CAD build for the part. Positions are in the model's coordinates, mm. A direction names the side the tool comes from. Coordinates: 2 decimals unless noted, no trailing zeros. Order: outer loops, then holes, each group sorted by start corner. A loop starts at its lowest first (then second) coordinate and runs counter-clockwise, first axis right, second up. Notation, with made-up numbers: (45, 83) - (93, 83) arc R15 cw to (93, 108) - close; hole circle Ø6 at (-1, 29). An arc over 180 degrees is marked (long way). Return JSON: item names as keys, results as strings.
from build123d import *

# Parameters (mm, degrees)
SKETCH1_R           = 5.55625
BOSS_EXTRUDE1_DEPTH = 12.7
BOSS_EXTRUDE2_DEPTH = 11.938


with BuildPart() as part:
    # Sketch1 → Boss-Extrude1 (new body)
    with BuildSketch(Plane(origin=(0, 0, 0), x_dir=(1, 0, 0), z_dir=(0, 1, 0))):
        Circle(SKETCH1_R)
    extrude(amount=BOSS_EXTRUDE1_DEPTH)

    # Sketch3 → Boss-Extrude2 (add)
    with BuildSketch(Plane(origin=(0, 12.7, 0), x_dir=(1, 0, 0), z_dir=(0, 1, 0))):
        Polygon((-10.287, 1.232393343), (-10.287, -1.232393343), (-6.210783894, -8.292606741), (-4.076216154, -9.525), (4.076216154, -9.525), (6.210783894, -8.292606741), (10.287, -1.232393343), (10.287, 1.232393343), (6.210783894, 8.292606741), (4.076216154, 9.525), (-4.076216154, 9.525), (-6.210783894, 8.292606741), align=None)
    extrude(amount=BOSS_EXTRUDE2_DEPTH)


solid = part.part
Item 1: Which spindle directions (+Z, -Z, +X, -X, +Y, -Y) get a long thin tool onto all of the face, cutting with end or side? Do faces 1 (the flat face through (-5, 12.7, -4)), 2 (the flat face through (0, 0, 0)). Say none if no direction does.
Findings below:
{"face 1": "-Y", "face 2": "+Z, -Z, +X, -X, -Y"}
Item 2: Band-saw the part on C-C, the plane x = 0. List the corners of the cut face in (y, z) (3 decimals).
Findings below:
{"outline": "(0, -5.556) - (12.7, -5.556) - (12.7, -9.525) - (24.638, -9.525) - (24.638, 9.525) - (12.7, 9.525) - (12.7, 5.556) - (0, 5.556) - close"}
Item 3: Band-saw the part on B-B, the plane y = 21.75. List the corners of the cut face in (x, z) (3 decimals).
Findings below:
{"outline": "(-10.287, -1.232) - (-6.211, -8.293) - (-4.076, -9.525) - (4.076, -9.525) - (6.211, -8.293) - (10.287, -1.232) - (10.287, 1.232) - (6.211, 8.293) - (4.076, 9.525) - (-4.076, 9.525) - (-6.211, 8.293) - (-10.287, 1.232) - close"}
Item 4: Band-saw the part on D-D, the plane y = 10.5. List the corners of the cut face in (x, z), then the cut area to 3 significant figures.
Findings below:
{"outline": "circle Ø11.11 at (0, 0)", "area": "97.0 mm²"}
Item 5: Drop flat-ended pins along their axis: P1, Ø6, axis at y = 12, z = -7.5, coming from the -X side; P2, Ø2, axis at x = -4, y = 3.5, coming from the -Z side; P3, Ø3, axis at x = -5, y = 10.5, coming from the +Z side. Give the stop position or say it passes through.
Findings below:
{"P1": "stops at x = -8.35", "P2": "stops at z = -4.68", "P3": "stops at z = 4.32"}
Item 6: Wall check: L1, parallel to Y at x = -1.5, z = 7.25; L2, parallel to X at y = 22.5, z = -1.25; L3, parallel to Z at x = -6.5, y = 21.75. Give the ranges that are in metal, low to high. Write a range as [from, to].
Findings below:
{"L1": "y = [12.7, 24.64]", "L2": "x = [-10.28, 10.28]", "L3": "z = [-7.79, 7.79]"}
Item 7: Band-saw the part on A-A, the plane z = 0. List the corners of the cut face in (x, y).
Findings below:
{"outline": "(-10.29, 12.7) - (-5.56, 12.7) - (-5.56, 0) - (5.56, 0) - (5.56, 12.7) - (10.29, 12.7) - (10.29, 24.64) - (-10.29, 24.64) - close"}
